Part model, mm, in its own coordinate system. A direction names the side the tool comes from. Give positions to 0.01 mm unless a question says otherwise; leave off trailing zeros. Write each loop counter-clockwise with the first axis right and the second up, starting at its lowest first coordinate (ties: lowest second). Pieces come first, ordered by that corner, then holes. Notation, with made-up numbers: M 23.25,84.25 L 61.25,84.25 A24 ccw 61.25,99.25 Z; hole C -16,70.5 d11. An arc over 180 degrees is marked long. Use a Markdown table: item, result.
```python
from build123d import *

# Parameters (mm, degrees)
PAD_DEPTH                          = 30
POCKET012_DEPTH                    = 28
POCKET013_DEPTH                    = 28
POCKET014_DEPTH                    = 18
FILLET005_R                        = 2
B_BOTTOM_CONNECTOR_ROLL_ANGLE      = 180
B_BOTTOM_CONNECTOR_PLACEMENT_ANGLE = 90


with BuildPart() as part:
    # Sketch039 → Pad (new body)
    with BuildSketch(Plane.XY):
        Polygon((5, 5), (13.5, 5), (13.5, -1.5), (-1.5, -1.5), (-1.5, 13.5), (5, 13.5), align=None)
    extrude(amount=PAD_DEPTH)

    # Sketch041 (on DatumPlane) → Pocket012 (cut)
    with BuildSketch(Plane.XY.offset(30)):
        Polygon((0, 10.1), (1.1, 10.1), (1.1, 1.1), (10.1, 1.1), (10.1, 0), (0, 0), align=None)
    extrude(amount=-POCKET012_DEPTH, mode=Mode.SUBTRACT)

    # Sketch040 (on X_Axis) → Pocket013 (cut)
    with BuildSketch(Plane.XY):
        Polygon((1, 11.1), (2.1, 11.1), (2.1, 2.1), (11.1, 2.1), (11.1, 1), (1, 1), align=None)
    extrude(amount=POCKET013_DEPTH, mode=Mode.SUBTRACT)

    # Sketch042 → Pocket014 (cut)
    with BuildSketch(Plane.XY):
        Polygon((2, 2.1), (3.1, 2.1), (3.1, 12.2), (-7, 12.2), (-7, 11.1), (2, 11.1), align=None)
    extrude(amount=POCKET014_DEPTH, mode=Mode.SUBTRACT)

    # Fillet005
    fillet005_edges = [part.edges().sort_by_distance(p)[0] for p in [
        (13.5, -1.5, 15),
        (-1.5, -1.5, 15),
        (13.5, 5, 15),
        (5, 13.5, 15),
    ]]
    fillet(fillet005_edges, radius=FILLET005_R)


with BuildPart() as part_1:
    # b_bottom_connector roll: moved
    add(part.part.rotate(Axis((0, 0, 0), (1, 0, 0)), B_BOTTOM_CONNECTOR_ROLL_ANGLE))


with BuildPart() as part_2:
    # b_bottom_connector placement: moved
    add(part_1.part.rotate(Axis((0, 0, 0), (0, 0, 1)), B_BOTTOM_CONNECTOR_PLACEMENT_ANGLE))


solid = part_2.part
```
1. Tool access for faces 1 (the flat face through (6, 1.1, -29)), 2 (the flat face through (0, 5, -16)), 3 (the flat face through (12.2, 1, -9)), 4 (the flat face through (2.1, 7, -14)), 5 (the flat face through (5, 8, -15)): list every direction of +Z, -Z, +X, -X, +Y, -Y with a clear straight run to the whole face (end or side of a thin tool).
Findings below:
| item | result |
|---|---|
| face 1 | +Z, -Z |
| face 2 | -Z |
| face 3 | +Z, -Y |
| face 4 | +Z |
| face 5 | +Z, -Z, +X, +Y |
2. Cut at B-B, the plane z = -22. Give the cut face in (x, y), then the cut area to 3 significant figures.
Findings below:
| item | result |
|---|---|
| outline | M -1.5,0.5 A2 ccw 0.5,-1.5 L 13.5,-1.5 L 13.5,3 A2 ccw 11.5,5 L 5,5 L 5,11.5 A2 ccw 3,13.5 L 0.5,13.5 A2 ccw -1.5,11.5 Z; hole M 0,0 L 10.1,0 L 10.1,1 L 11.1,1 L 11.1,2.1 L 2.1,2.1 L 2.1,11.1 L 1,11.1 L 1,10.1 L 0,10.1 Z |
| area | 109 mm2 |
3. Drill centre lines: L1, parallel to X at y = 1.25, z = -10; L2, parallel to X at y = 8.25, z = -23; L3, parallel to Y at x = 2, z = -7.25. Where is each one in solid material? Low to high.
Findings below:
| item | result |
|---|---|
| L1 | -1.5 to 0, 12.2 to 13.5 |
| L2 | -1.5 to 0, 2.1 to 5 |
| L3 | -1.5 to 0, 11.1 to 13.5 |
4. Drop flat-ended pins along their axis: P1, Ø2, axis at y = 9, z = -13, coming from the +X side; P2, Ø5, axis at x = 8.5, z = -13, coming from the +Y side; P3, Ø8, axis at x = 8.5, z = -24.5, coming from the +Y side. Give the stop position or say it passes through.
Findings below:
| item | result |
|---|---|
| P1 | x = 5 |
| P2 | y = 5 |
| P3 | y = 12.82 |
5. Cut at A-A, the plane x = 1.5. Give the cut face in (y, z).
Findings below:
| item | result |
|---|---|
| outline | M -1.5,-30 L 0,-30 L 0,-2 L 1,-2 L 1,0 L -1.5,0 Z; M 1.1,-30 L 13.5,-30 L 13.5,0 L 11.1,0 L 11.1,-28 L 1.1,-28 Z |
6. Two-plate mould, pull along Y, no slides. Class faces 6 (the cylindrical face through (12.93, 4.4, -15.21)), 7 (the flat face through (11.1, 1.5, -22.9)), 8 (the flat face through (-1.5, 6, -15)), 9 (the flat face through (8.3, 2.5, -18)): released by +Y, released by -Y, zero draft, split by the parting line, or undercut.
Findings below:
| item | result |
|---|---|
| face 6 | released by +Y |
| face 7 | undercut |
| face 8 | zero draft |
| face 9 | undercut |
7. Cut at D-D, the plane z = -3.75. Give the cut face in (x, y), then the cut area to 3 significant figures.
Findings below:
| item | result |
|---|---|
| outline | M -1.5,0.5 A2 ccw 0.5,-1.5 L 11.1,-1.5 L 11.1,1 L 10.1,1 L 10.1,0 L 0,0 L 0,10.1 L 1,10.1 L 1,11.1 L 2.1,11.1 L 2.1,3.1 L 12.2,3.1 L 12.2,-1.5 L 13.5,-1.5 L 13.5,3 A2 ccw 11.5,5 L 5,5 L 5,11.5 A2 ccw 3,13.5 L 0.5,13.5 A2 ccw -1.5,11.5 Z |
| area | 95.0 mm2 |
8. Cut at C-C, the plane x = 10.5. Give the cut face in (y, z), then the cut area to 3 significant figures.
Findings below:
| item | result |
|---|---|
| outline | M -1.5,-30 L 5,-30 L 5,0 L 3.1,0 L 3.1,-18 L 2.1,-18 L 2.1,-28 L 1,-28 L 1,0 L -1.5,0 Z |
| area | 146 mm2 |
